from build123d import *

# Parameters (mm, degrees)
SKETCH1_R          = 60
SKETCH1_R_2        = 43.5
EXTRUSION1_DEPTH   = 60
EXTRUSION3_START   = -60
EXTRUSION3_DEPTH   = 60
CUT_EXTRUDE2_DEPTH = 55
CUT_EXTRUDE3_DEPTH = 10
CUT_EXTRUDE4_DEPTH = 35
CUT_EXTRUDE5_DEPTH = 104.923048454
CUT_EXTRUDE6_DEPTH = 30
CUT_EXTRUDE7_DEPTH = 30


with BuildPart() as part:
    # Sketch1 → Extrusion1 (new body)
    with BuildSketch(Plane.XY):
        Circle(SKETCH1_R)
        Circle(SKETCH1_R_2, mode=Mode.SUBTRACT)
    extrude(amount=EXTRUSION1_DEPTH)

    # Sketch3 → Extrusion3 (cut)
    with BuildSketch(Plane.XY.offset(60).offset(EXTRUSION3_START)):
        with BuildLine():
            Line((-0.5, 48.5), (-0.5, 43.497126342))
            ThreePointArc((-0.5, 43.497126342), (0, 43.5), (0.5, 43.497126342))
            Line((0.5, 43.497126342), (0.5, 48.5))
            Line((0.5, 48.5), (-0.5, 48.5))
        make_face()
    extrude(amount=EXTRUSION3_DEPTH, mode=Mode.SUBTRACT)

    # Sketch4 → Cut-Extrude2 (cut)
    with BuildSketch(Plane(origin=(0, 0, 0), x_dir=(-1, 0, 0), z_dir=(0, 0, -1))):
        with BuildLine():
            ThreePointArc((-50.316139758, -0.506318633), (-49.782828126, -7.323954021), (-48.330045697, -14.006318633))
            Line((-48.330045697, -14.006318633), (-46.316139758, -14.006318633))
            ThreePointArc((-46.316139758, -14.006318633), (-45.609032977, -13.713425414), (-45.316139758, -13.006318633))
            Line((-45.316139758, -13.006318633), (-45.316139758, 11.993681367))
            ThreePointArc((-45.316139758, 11.993681367), (-45.609032977, 12.700788148), (-46.316139758, 12.993681367))
            Line((-46.316139758, 12.993681367), (-54.316139758, 12.993681367))
            ThreePointArc((-54.316139758, 12.993681367), (-55.023246539, 12.700788148), (-55.316139758, 11.993681367))
            Line((-55.316139758, 11.993681367), (-55.316139758, -0.506318633))
            Line((-55.316139758, -0.506318633), (-50.316139758, -0.506318633))
        make_face()
        with BuildLine():
            Line((-54.316139758, -14.006318633), (-48.330045697, -14.006318633))
            ThreePointArc((-48.330045697, -14.006318633), (-49.782828126, -7.323954021), (-50.316139758, -0.506318633))
            Line((-50.316139758, -0.506318633), (-55.316139758, -0.506318633))
            Line((-55.316139758, -0.506318633), (-55.316139758, -13.006318633))
            ThreePointArc((-55.316139758, -13.006318633), (-55.023246539, -13.713425414), (-54.316139758, -14.006318633))
        make_face()
        with BuildLine():
            Line((55.316139758, 0), (50.318687172, 0))
            ThreePointArc((50.318687172, 0), (49.819046203, -7.07339481), (48.330045697, -14.006318633))
            Line((48.330045697, -14.006318633), (54.316139758, -14.006318633))
            ThreePointArc((54.316139758, -14.006318633), (55.023246539, -13.713425414), (55.316139758, -13.006318633))
            Line((55.316139758, -13.006318633), (55.316139758, 0))
        make_face()
        with BuildLine():
            ThreePointArc((48.330045697, -14.006318633), (49.819046203, -7.07339481), (50.318687172, 0))
            Line((50.318687172, 0), (55.316139758, 0))
            Line((55.316139758, 0), (55.316139758, 11.993681367))
            ThreePointArc((55.316139758, 11.993681367), (55.023246539, 12.700788148), (54.316139758, 12.993681367))
            Line((54.316139758, 12.993681367), (46.316139758, 12.993681367))
            ThreePointArc((46.316139758, 12.993681367), (45.609032977, 12.700788148), (45.316139758, 11.993681367))
            Line((45.316139758, 11.993681367), (45.316139758, -13.006318633))
            ThreePointArc((45.316139758, -13.006318633), (45.609032977, -13.713425414), (46.316139758, -14.006318633))
            Line((46.316139758, -14.006318633), (48.330045697, -14.006318633))
        make_face()
    extrude(amount=-CUT_EXTRUDE2_DEPTH, mode=Mode.SUBTRACT)

    # Sketch5 → Cut-Extrude3 (cut)
    with BuildSketch(Plane(origin=(0, 0, 0), x_dir=(-1, 0, 0), z_dir=(0, 0, -1))):
        with BuildLine():
            Line((-52.51879057, -14.006318633), (-48.51879057, -14.006318633))
            ThreePointArc((-48.51879057, -14.006318633), (0, -50.5), (48.51879057, -14.006318633))
            Line((48.51879057, -14.006318633), (51.634029848, -14.006318633))
            ThreePointArc((51.634029848, -14.006318633), (-0.442380361, -55.246730559), (-52.51879057, -14.006318633))
        make_face()
    extrude(amount=-CUT_EXTRUDE3_DEPTH, mode=Mode.SUBTRACT)

    # Sketch7 → Cut-Extrude4 (cut)
    with BuildSketch(Plane(origin=(0, 0, 0), x_dir=(-1, 0, 0), z_dir=(0, 0, -1))):
        with BuildLine():
            Line((21.085956356, -51.080456264), (42.59953536, -36.48025358))
            ThreePointArc((42.59953536, -36.48025358), (43.020154485, -35.840827283), (42.865434449, -35.091261977))
            Line((42.865434449, -35.091261977), (39.496156907, -30.126589899))
            ThreePointArc((39.496156907, -30.126589899), (38.856730609, -29.705970774), (38.107165303, -29.860690809))
            Line((38.107165303, -29.860690809), (16.593586299, -44.460893494))
            ThreePointArc((16.593586299, -44.460893494), (16.172967174, -45.100319791), (16.32768721, -45.849885097))
            Line((16.32768721, -45.849885097), (19.696964752, -50.814557175))
            ThreePointArc((19.696964752, -50.814557175), (20.33639105, -51.2351763), (21.085956356, -51.080456264))
        make_face()
    extrude(amount=-CUT_EXTRUDE4_DEPTH, mode=Mode.SUBTRACT)

    # Sketch8 → Cut-Extrude5 (cut, through all)
    with BuildSketch(Plane(origin=(0, 0, 0), x_dir=(-1, 0, 0), z_dir=(0, 0, -1))):
        with BuildLine():
            Line((0, -54.348403173), (0, -51.348403173))
            Line((0, -51.348403173), (-4, -51.348403173))
            ThreePointArc((-4, -51.348403173), (-4.707106781, -51.641296392), (-5, -52.348403173))
            Line((-5, -52.348403173), (-5, -53.348403173))
            ThreePointArc((-5, -53.348403173), (-4.707106781, -54.055509954), (-4, -54.348403173))
            Line((-4, -54.348403173), (0, -54.348403173))
        make_face()
        with BuildLine():
            Line((4, -51.348403173), (0, -51.348403173))
            Line((0, -51.348403173), (0, -54.348403173))
            Line((0, -54.348403173), (4, -54.348403173))
            ThreePointArc((4, -54.348403173), (4.707106781, -54.055509954), (5, -53.348403173))
            Line((5, -53.348403173), (5, -52.348403173))
            ThreePointArc((5, -52.348403173), (4.707106781, -51.641296392), (4, -51.348403173))
        make_face()
    extrude(amount=-CUT_EXTRUDE5_DEPTH, mode=Mode.SUBTRACT)

    # Sketch9 → Cut-Extrude6 (cut)
    with BuildSketch(Plane(origin=(0, 0, 0), x_dir=(-1, 0, 0), z_dir=(0, 0, -1))):
        with BuildLine():
            Line((-46.541704455, -20.656628598), (-48.174808597, -21.811172171))
            ThreePointArc((-48.174808597, -21.811172171), (-50.216361173, -25.047948966), (-49.371210022, -28.780291457))
            Line((-49.371210022, -28.780291457), (-43.598492159, -36.945812168))
            ThreePointArc((-43.598492159, -36.945812168), (-40.361715364, -38.987364744), (-36.629372873, -38.142213593))
            Line((-36.629372873, -38.142213593), (-34.996268731, -36.98767002))
            ThreePointArc((-34.996268731, -36.98767002), (-32.954716155, -33.750893225), (-33.799867306, -30.018550734))
            Line((-33.799867306, -30.018550734), (-39.572585168, -21.853030023))
            ThreePointArc((-39.572585168, -21.853030023), (-42.809361964, -19.811477447), (-46.541704455, -20.656628598))
        make_face()
    extrude(amount=-CUT_EXTRUDE6_DEPTH, mode=Mode.SUBTRACT)

    # Sketch10 → Cut-Extrude7 (cut)
    with BuildSketch(Plane(origin=(0, 0, 0), x_dir=(-1, 0, 0), z_dir=(0, 0, -1))):
        with BuildLine():
            Line((-16.862196749, -52.664700174), (-15.619636194, -50.065338059))
            Line((-15.619636194, -50.065338059), (-29.152890755, -43.596101551))
            Line((-29.152890755, -43.596101551), (-30.352191828, -46.104967426))
            ThreePointArc((-30.352191828, -46.104967426), (-23.838237424, -49.859970652), (-16.862196749, -52.664700174))
        make_face()
        with BuildLine():
            Line((-16.913483495, -52.771988971), (-16.862196749, -52.664700174))
            ThreePointArc((-16.862196749, -52.664700174), (-23.838237424, -49.859970652), (-30.352191828, -46.104967426))
            Line((-30.352191828, -46.104967426), (-30.446738056, -46.302752463))
            ThreePointArc((-30.446738056, -46.302752463), (-30.487447557, -47.067035901), (-29.975803519, -47.636251867))
            Line((-29.975803519, -47.636251867), (-18.2469829, -53.242923508))
            ThreePointArc((-18.2469829, -53.242923508), (-17.482699462, -53.283633009), (-16.913483495, -52.771988971))
        make_face()
        with BuildLine():
            ThreePointArc((-28.304856483, -41.822064744), (-21.77976291, -45.561957021), (-14.771601922, -48.291301252))
            Line((-14.771601922, -48.291301252), (-14.325788892, -47.358687147))
            ThreePointArc((-14.325788892, -47.358687147), (-14.285079391, -46.594403708), (-14.796723429, -46.025187742))
            Line((-14.796723429, -46.025187742), (-26.525544048, -40.418516102))
            ThreePointArc((-26.525544048, -40.418516102), (-27.289827487, -40.377806601), (-27.859043453, -40.889450639))
            Line((-27.859043453, -40.889450639), (-28.304856483, -41.822064744))
        make_face()
        with BuildLine():
            Line((-29.152890755, -43.596101551), (-15.619636194, -50.065338059))
            Line((-15.619636194, -50.065338059), (-14.771601922, -48.291301252))
            ThreePointArc((-14.771601922, -48.291301252), (-21.77976291, -45.561957021), (-28.304856483, -41.822064744))
            Line((-28.304856483, -41.822064744), (-29.152890755, -43.596101551))
        make_face()
    extrude(amount=-CUT_EXTRUDE7_DEPTH, mode=Mode.SUBTRACT)


solid = part.part
Check sheet for the modelled part. Datum: model origin and axes. Units: mm. A direction names the side the tool comes from. Give positions to 0.01 mm unless a question says otherwise; leave off trailing zeros. Write each loop counter-clockwise with the first axis right and the second up, starting at its lowest first coordinate (ties: lowest second). Pieces come first, ordered by that corner, then holes. Notation, with made-up numbers: (-4.75, -40) -> (15.25, -40) arc R23 ccw to (15.25, -10) -> close; hole circle Ø7 at (-26.75, 3). An arc over 180 degrees is marked (long way). Write item = value, one per line.
Item 1: Release check for a two-part mould opening along X. For faces 1 (the flat face through (-18, 40, 0)), 2 (the flat face through (-46, -24, 10)) record: +X half, -X half, draft (parallel to the pull), parting line (faces both ways), or undercut.
Output:
face_1 = draft
face_2 = undercut
Item 2: Sectioned sample at B-B on y = -5.5. Record the boundary of the cut face in (x, z), and give its area (3 significant figures).
Output:
outline = (-59.75, 0) -> (-55.32, 0) -> (-55.32, 55) -> (-45.32, 55) -> (-45.32, 0) -> (-43.15, 0) -> (-43.15, 60) -> (-59.75, 60) -> close; (43.15, 0) -> (45.32, 0) -> (45.32, 55) -> (55.32, 55) -> (55.32, 0) -> (59.75, 0) -> (59.75, 60) -> (43.15, 60) -> close
area = 892 mm^2
Item 3: Scan lines: probe 1 along Y at (x, z) = (0, 28); probe 2 along X at (y, z) = (-51.5, 19.5); probe 3 along Y at (x, z) = (-32, 24). Record each from-to range of solid material in increasing order. Write a range as from..to.
Output:
probe_1 = -60..-54.35, -51.35..-43.5, 48.5..60
probe_2 = -30.79..-4.53, 4.53..16.31, 21.89..30.79
probe_3 = -50.75..-43.67, -34.01..-29.47, 29.47..50.75
Item 4: Sectioned sample at A-A on z = 41.5. Count the separate pieces of the cut face and the enclosed holes in it, and give its area (3 significant figures).
Output:
separate_pieces = 1
enclosed_holes = 4
area = 4,790 mm^2
Item 5: Gauge pin test, flat ends, axial feed: pin 1 (3 mm diameter, centred on y = 43, z = 52, fed in from -X); pin 2 (12 mm diameter, centred on x = -10, y = 33, fed in from +Z); pin 3 (3 mm diameter, centred on x = 49.5, y = 0, fed in from -Z); pin 4 (2.5 mm diameter, centred on x = 50.5, z = 18, fed in from +Y). Record the tip position at first contact, or that the pin passes through.
Output:
pin_1 = -43.33
pin_2 = through
pin_3 = 55
pin_4 = 34.27
Item 6: Sectioned sample at D-D on y = 14.5. Record the boundary of the cut face in (x, z).
Output:
outline = (-58.22, 0) -> (-41.01, 0) -> (-41.01, 60) -> (-58.22, 60) -> close; (41.01, 0) -> (58.22, 0) -> (58.22, 60) -> (41.01, 60) -> close
Item 7: Tool access check on faces 3 (the flat face through (17.5, 40.3, 60)), 4 (the flat face through (0, -51.348, 35)), 5 (the flat face through (50, 12.994, 27)). Record the directions out of +Z, -Z, +X, -X, +Y, -Y that give a thin tool (end or side, any length) a straight path to the whole face; none if there is none.
Output:
face_3 = +Z, +X, -X, +Y, -Y
face_4 = +Z, -Z
face_5 = -Z
Item 8: Sectioned sample at C-C on x = -13. Record the boundary of the cut face in (y, z), and give its area (3 significant figures).
Output:
outline = (-58.57, 0) -> (-53.53, 0) -> (-53.53, 10) -> (-48.8, 10) -> (-48.8, 0) -> (-41.51, 0) -> (-41.51, 60) -> (-58.57, 60) -> close; (41.51, 0) -> (58.57, 0) -> (58.57, 60) -> (41.51, 60) -> close
area = 2,000 mm^2
